The listing builds one solid part. Answer for the finished solid, in the listing's coordinates (mm). A direction names the side the tool comes from. Round coordinates to 2 decimals unless told otherwise and drop trailing zeros. Order: outer loops, then holes, each group sorted by start corner. A loop starts at its lowest first (then second) coordinate and runs counter-clockwise, first axis right, second up. Notation, with made-up numbers: (-13, 77) - (29, 77) arc R20 cw to (29, 116) - close; hole circle Ø10 at (16.25, 14.25). An arc over 180 degrees is marked (long way). One line per item, written item: value. Start each with the question number.
1. Section C-C, the plane x = -44 is taken. Give the vertices of the cut face in (y, z), then the cut area to 3 significant figures.
2. Straight lines are drawn through the part: line 1 (Y direction, x = -44, z = 41.35); line 2 (X direction, y = -19, z = 31.5); line 3 (Z direction, x = 12.5, y = 16). For each, find the intervals that lie inside material, in ascending order.
3. Flat-ended cylindrical pins translate along their axes: P1, Ø2, axis at y = 8.5, z = 4.5, coming from the -X side; P2, Ø10, axis at y = 15, z = 7, coming from the +X side; P3, Ø1, axis at x = 7, y = 8, coming from the +Z side. Find the tip coordinate at first contact, or state that the pin passes through.
4. Section A-A, the plane z = 29.5 is taken. Give the vertices of the cut face in (x, y).
5. Section D-D, the plane y = -12 is taken. Give the vertices of the cut face in (x, z), then the cut area to 3 significant figures.
6. A tool of negligible diameter and unlimited length cuts with its end or side. For faces 1 (the flat face through (44, 7.5, 42)), 2 (the flat face through (-1, -24, 23)), 3 (the flat face through (1, -22.5, 11)), 4 (the flat face through (47, 2, 40)), 5 (the flat face through (44, -7.5, 42)), from which of +Z, -Z, +X, -X, +Y, -Y can it reach the whole face along a straight path? Write none if from no direction.
7. For a pull along X with two mould halves and no side action, classify faces 6 (the flat face through (36, 0, 21)), 7 (the flat face through (40, 8.5, 41.1)), 8 (the flat face through (1, 0, -3)) as released by +X, released by -X, zero draft, split by the parting line, or undercut.
8. Section B-B, the plane y = 0 is taken. Give the vertices of the cut face in (x, z), then the cut area to 3 significant figures.
Autodesk Inventor part; units mm, degrees
ref_plane "YZ Plane" through (0, 0, 0) normal (1, 0, 0) x (0, 1, 0)
ref_plane "XZ Plane" through (0, 0, 0) normal (0, 1, 0) x (-1, 0, 0)
ref_plane "XY Plane" through (0, 0, 0) normal (0, 0, 1) x (1, 0, 0)
sketch "Sketch1" plane through (0, 0, 0) normal (0, 0, 1) x (1, 0, 0)
  line L0 (-36, 22.5) -> (36, 22.5)
  line L1 (36, 22.5) -> (36, -22.5)
  line L2 (36, -22.5) -> (-36, -22.5)
  line L3 (-36, -22.5) -> (-36, 22.5)
  line L4 (-36, 22.5) -> (36, -22.5) construction
  line L5 (36, 22.5) -> (-36, -22.5) construction
  line L6 (39, 25.5) -> (-39, 25.5)
  line L7 (-39, 25.5) -> (-39, -25.5)
  line L8 (-39, -25.5) -> (39, -25.5)
  line L9 (39, -25.5) -> (39, 25.5)
  point P0 (0, 0)
  dimension "d0" = 72
  dimension "d1" = 45
  dimension "d2" = 3
extrude "Extrusion1" add sketch "Sketch1" along normal blind 43
sketch "Sketch2" plane through (0, 0, 0) normal (0, 0, -1) x (-1, 0, 0)
  line L0 (-39, 25.5) -> (39, 25.5)
  line L1 (39, 25.5) -> (39, -25.5)
  line L2 (-39, 25.5) -> (39, 25.5)
  line L3 (39, 25.5) -> (39, -25.5)
  line L4 (39, -25.5) -> (-39, -25.5)
  line L5 (-39, -25.5) -> (-39, 25.5)
  point P0 (0, 0)
extrude "Extrusion2" add sketch "Sketch2" along normal blind 3
sketch "Sketch3" plane through (-39, 25.5, 43) normal (0, 1, 0) x (1, 0, 0)
  line L0 (3, 43) -> (75, 43)
  line L1 (75, 43) -> (75, 0)
  line L2 (3, 43) -> (75, 43)
  line L3 (75, 43) -> (75, 0)
  line L4 (75, 0) -> (3, 0)
  line L5 (3, 0) -> (3, 43)
  point P0 (39, 43)
extrude "Extrusion3" cut sketch "Sketch3" against normal up to surface (3 mm away)
ref_plane "Work Plane1" through (0, -25.5, 43) normal (-1, 0, 0) x (0, 0, 1)
sketch "Sketch5" plane through (0, 0, 43) normal (0, 0, 1) x (1, 0, 0)
  line L0 (-39, -25.5) -> (-39, 25.5)
  line L1 (-39, 7.5) -> (-47, 7.5)
  line L2 (-49, 5.5) -> (-49, -5.5)
  line L3 (-47, -7.5) -> (-39, -7.5)
  line L4 (-39, -7.5) -> (-39, 7.5)
  line L5 (-36, 25.5) -> (-39, 25.5)
  circle A0 centre (-44, 0) radius 2.75
  arc A1 (-49, -5.5) -> (-47, -7.5) centre (-47, -5.5) ccw
  arc A2 (-47, 7.5) -> (-49, 5.5) centre (-47, 5.5) ccw
  point P0 (0, 0)
  point P1 (-49, -7.5)
  point P2 (-49, 7.5)
  dimension "d12" = 10
  dimension "d13" = 15
  dimension "d14" = 18
  dimension "d17" = 5.5
  dimension "d18" = 5
  dimension "d21" = 2
extrude "Extrusion5" add sketch "Sketch5" against normal blind 3
mirror "Mirror1" about plane through (0, -25.5, 43) normal (-1, 0, 0) of "Extrusion5"
chamfer "Chamfer1" distance 2 angle 45 6 edges at (-39, 0, 40) (-39, 7.5, 41.5) (-39, -7.5, 41.5) (39, 0, 40) (39, -7.5, 41.5) (39, 7.5, 41.5)
fillet "Fillet1" radius 2 8 edges at (39, 0, -3) (-39, 0, -3) (-39, -25.5, 20) (0, -25.5, -3) (39, -25.5, 20) (0, 25.5, -3) (-37.5, 25.5, 43) (37.5, 25.5, 43)
sketch "Sketch7" plane through (-37, -25.5, -1) normal (0, -1, 0) x (1, 0, 0)
  line L0 (73, 44) -> (1, 44)
  line L1 (1, 1) -> (1, 44)
  line L2 (73, 44) -> (1, 44)
  line L3 (1, 44) -> (1, 24)
  line L4 (1, 24) -> (73, 24)
  line L5 (73, 24) -> (73, 44)
  point P0 (37, 1)
  dimension "d26" = 20
extrude "Extrusion6" cut sketch "Sketch7" against normal up to surface (3 mm away)
equation "\"d18\" = 0.5 * d12"
properties part number "Eletronica - protecaoFonte"
Answer list:
1. outline: (-7.5, 40) - (-2.75, 40) - (-2.75, 43) - (-7.5, 43) - close; (2.75, 40) - (7.5, 40) - (7.5, 43) - (2.75, 43) - close
1. area: 28.5 mm²
2. line 1: y = -7.5 to -2.75, 2.75 to 7.5
2. line 2: x = -39 to -36, 36 to 39
2. line 3: z = -3 to 0
3. P1: stops at x = -39
3. P2: stops at x = 39
3. P3: stops at z = 0
4. outline: (-39, -23.5) arc R2 ccw to (-37, -25.5) - (-36, -25.5) - (-36, 25.5) - (-39, 25.5) - close; (36, -25.5) - (37, -25.5) arc R2 ccw to (39, -23.5) - (39, 25.5) - (36, 25.5) - close
5. outline: (-39, -1) arc R2 ccw to (-37, -3) - (37, -3) arc R2 ccw to (39, -1) - (39, 43) - (36, 43) - (36, 0) - (-36, 0) - (-36, 43) - (-39, 43) - close
5. area: 490 mm²
6. face 1: +Z, -Z, +X, +Y
6. face 2: +Z, +Y, -Y
6. face 3: +Z, +Y
6. face 4: -Z, +X, +Y, -Y
6. face 5: +Z, -Z, +X, -Y
7. face 6: undercut
7. face 7: released by +X
7. face 8: zero draft
8. outline: (-49, 40) - (-46.75, 40) - (-46.75, 43) - (-49, 43) - close; (-41.25, 40) - (-41, 40) - (-39, 38) - (-39, -1) arc R2 ccw to (-37, -3) - (37, -3) arc R2 ccw to (39, -1) - (39, 38) - (41, 40) - (41.25, 40) - (41.25, 43) - (36, 43) - (36, 0) - (-36, 0) - (-36, 43) - (-41.25, 43) - close; (46.75, 40) - (49, 40) - (49, 43) - (46.75, 43) - close
8. area: 521 mm²
